Design review of the part built by this model. Coordinates are the model's own, in mm. A direction names the side the tool comes from. Round coordinates to 2 decimals unless told otherwise and drop trailing zeros. Write each loop counter-clockwise with the first axis right and the second up, starting at its lowest first coordinate (ties: lowest second). Pieces come first, ordered by that corner, then holes. Notation, with made-up numbers: (78.5, 86) -> (97.5, 86) arc R22 cw to (97.5, 102) -> close; hole circle Ø2 at (-35.75, -40). An arc over 180 degrees is marked (long way). Write item = value, one per line. Start each with the question number.
Item 1: Add section A-A, the plane y = 39. State the section outline as (x, z) points (3 decimals), then the cut area to 3 significant figures.
Item 2: For pin 1 Ø1 at (x, z) = (-23.5, 14) entering from -Y; pin 2 Ø16 at (x, y) = (-10, -34) entering from +Z (3 decimals); pin 3 Ø4 at (y, z) = (-13.5, 21.5) entering from +X (3 decimals), all flat-tipped, find the tip position at first contact; note any pin that passes through.
Item 3: Add section B-B, the plane y = -30.5. State the section outline as (x, z) points (3 decimals).
Item 4: To check wall thickness, follow L1, parallel to Z at x = 3.5, y = -39 (3 decimals); L2, parallel to X at y = -44.5, z = 0.5 (3 decimals); L3, parallel to Y at x = 7, z = 22.5. State the ranges of each line that lie inside material, in increasing order.
Item 5: Mouldability with a two-part tool opening along X and no side actions: class faces 6 (the flat face through (-1, -1, -9.525)), 7 (the flat face through (60, 2, 42.875)), 8 (the cylindrical face through (39.8, -62, -1.2)) as released by +X, released by -X, zero draft, split by the parting line, or undercut.
Item 6: Machinability: for faces 1 (the flat face through (60, -2, 61.925)), 2 (the flat face through (46, 25.4, 42)), 3 (the flat face through (86, 0, 38.1)), 4 (the cylindrical face through (-39.8, 62, -0.1)), 5 (the flat face through (22.225, 17, 18)), which of the approach directions +Z, -Z, +X, -X, +Y, -Y give a long, thin tool a straight path to every point of the face, cutting with its end or side? Answer none if there is none.
from build123d import *

# Parameters (mm, degrees)
F1_DEPTH     = 63.5
F0_W         = 25.4
F0_H         = 19.05
F2_DEPTH     = 25.4
F3_DEPTH     = 7.9375
F5_R         = 5.08
F6_T1_DEPTH  = 72.39
F6_T3_DEPTH  = 33.02
F6_T5_DEPTH  = 50.4825
F6_T10_ANGLE = 90
F6_T12_ANGLE = 90


# Not quite as in the source:
# - a fillet or chamfer that OpenCascade refuses, or shapes differently, is made with other operations: its cross-section is extruded or revolved along the edge and cut away or added


with BuildPart() as f1:
    # F0 (on Front) → F1 (new body, symmetric)
    with BuildSketch(Plane.XZ):
        Polygon((22.225, 9.525), (-41.275, 9.525), (-41.275, -9.525), (41.275, -9.525), (41.275, 9.525), align=None)
    extrude(amount=F1_DEPTH, both=True)

    # F0 (on Front) → F2 (join, symmetric)
    with BuildSketch(Plane.XZ):
        with BuildLine():
            Line((22.225, 27.0002), (22.225, 9.525))
            Line((22.225, 9.525), (41.275, 9.525))
            Line((41.275, 9.525), (41.275, 27.0002))
            ThreePointArc((41.275, 27.0002), (45.9246798487, 38.2255201513), (57.15, 42.8752))
            Line((57.15, 42.8752), (60.325, 42.8752))
            Line((60.325, 42.8752), (60.325, 61.9252))
            Line((60.325, 61.9252), (57.15, 61.9252))
            add(Edge.make_bspline(
                [(53.8854342407, 61.7722898912), (54.9842067368, 61.8365871986), (56.0728453275, 61.8876096574), (57.15, 61.9252)],
                knots=[108.5245810491, 108.5245810491, 108.5245810491, 108.5245810491, 111.5045361635, 111.5045361635, 111.5045361635, 111.5045361635], degree=3))
            ThreePointArc((53.8854342407, 61.7722898912), (31.3258777096, 50.5133948686), (22.225, 27.0002))
        make_face()
        with Locations((73.025, 52.4002)):
            Rectangle(F0_W, F0_H)
    extrude(amount=F2_DEPTH, both=True)

    # F0 (on Front) → F3 (join, symmetric)
    with BuildSketch(Plane.XZ):
        with BuildLine():
            add(Edge.make_bspline(
                [(-41.275, 9.525), (-39.5856284224, 39.4828766469), (13.870125209, 59.4306981306), (53.8854342407, 61.7722898912)],
                knots=[0, 0, 0, 0, 108.5245810491, 108.5245810491, 108.5245810491, 108.5245810491], degree=3))
            Line((-41.275, 9.525), (22.225, 9.525))
            Line((22.225, 9.525), (22.225, 27.0002))
            ThreePointArc((22.225, 27.0002), (31.3258777096, 50.5133948686), (53.8854342407, 61.7722898912))
        make_face()
    extrude(amount=F3_DEPTH, both=True)

    # F0 (on Front) → F4 (revolve)
    with BuildSketch(Plane.XZ):
        Polygon((85.725, 66.675), (85.725, 61.9252), (85.725, 42.8752), (85.725, 38.1), (111.125, 38.1), (111.125, 66.675), align=None)
    revolve(axis=Axis((85.725, 0, 52.3875), (0, 0, 1)))

    # F5
    f5_edges = [f1.edges().sort_by_distance(p)[0] for p in [
        (41.275, -63.5, 0),
        (-41.275, -63.5, 0),
        (41.275, 63.5, 0),
        (-41.275, 63.5, 0),
    ]]
    fillet(f5_edges, radius=F5_R)

    # F6: chamfer of 2.54 on 6 edges, made by hand

    # F6_s2 → F6_t1 (cut)
    with BuildSketch(Plane.YZ.offset(-36.195)):
        Polygon((-60.96, 9.525), (-63.5, 6.985), (-63.5, 9.525), align=None)
    extrude(amount=F6_T1_DEPTH, mode=Mode.SUBTRACT)

    # F6_s4 → F6_t3 (cut)
    with BuildSketch(Plane.XZ.offset(25.4)):
        Polygon((41.275, 6.985), (38.735, 9.525), (41.275, 9.525), align=None)
    extrude(amount=F6_T3_DEPTH, mode=Mode.SUBTRACT)

    # F6_s6 → F6_t5 (cut)
    with BuildSketch(Plane.XZ.offset(7.9375)):
        Polygon((-41.275, 6.985), (-38.735, 9.525), (-41.275, 9.525), align=None)
    extrude(amount=F6_T5_DEPTH, mode=Mode.SUBTRACT)

    # F6_s7 → F6_t8 (revolve, cut)
    with BuildSketch(Plane.XZ):
        Polygon((111.125, 64.135), (108.585, 66.675), (111.125, 66.675), align=None)
    revolve(axis=Axis((85.725, 0, 66.675), (0, 0, 1)), mode=Mode.SUBTRACT)

    # F6_s9 → F6_t10 (revolve, cut)
    with BuildSketch(Plane.XZ.offset(58.42)):
        Polygon((41.275, 6.985), (38.735, 9.525), (41.275, 9.525), align=None)
    revolve(axis=Axis((36.195, -58.42, 9.525), (0, 0, -1)), revolution_arc=F6_T10_ANGLE, mode=Mode.SUBTRACT)

    # F6_s11 → F6_t12 (revolve, cut)
    with BuildSketch(Plane.XZ.offset(58.42)):
        Polygon((-38.735, 9.525), (-41.275, 6.985), (-41.275, 9.525), align=None)
    revolve(axis=Axis((-36.195, -58.42, 9.525), (0, 0, 1)), revolution_arc=F6_T12_ANGLE, mode=Mode.SUBTRACT)


solid = f1.part
Result set:
q1.outline = (-41.275, -9.525) -> (41.275, -9.525) -> (41.275, 9.525) -> (-41.275, 9.525) -> close
q1.area = 1,570 mm²
q2.pin_1 = -7.94
q2.pin_2 = 9.525
q2.pin_3 = 41.275
q3.outline = (-41.275, -9.525) -> (41.275, -9.525) -> (41.275, 6.985) -> (38.735, 9.525) -> (-38.735, 9.525) -> (-41.275, 6.985) -> close
q4.L1 = -9.525 to 9.525
q4.L2 = -41.275 to 41.275
q4.L3 = -7.94 to 7.94
q5.face_6 = zero draft
q5.face_7 = undercut
q5.face_8 = released by +X
q6.face_1 = +Z, -X
q6.face_2 = +Z, +X, -X, +Y
q6.face_3 = -Z, +X, +Y, -Y
q6.face_4 = +Z, -Z, -X, +Y
q6.face_5 = +Z, -X, +Y
